```python
from build123d import *

# Parameters (mm, degrees)
F0_R     = 40.1
F1_DEPTH = 10
F2_R     = 38.1
F3_DEPTH = 8
F4_R     = 0.99999


# Not quite as in the source:
# - a fillet or chamfer is up to 0.001 mm smaller than in the source, because OpenCascade refuses the exact size


with BuildPart() as f1:
    # F0 (on Top) → F1 (new body)
    with BuildSketch(Plane.XY):
        Circle(F0_R)
    extrude(amount=F1_DEPTH)

    # F2 (on face) → F3 (cut)
    with BuildSketch(Plane.XY.offset(10)):
        Circle(F2_R)
    extrude(amount=-F3_DEPTH, mode=Mode.SUBTRACT)

    # F4 (radius 1 in the source; OpenCascade refuses exactly that, so slightly less here)
    f4_edges = [f1.edges().sort_by_distance(p)[0] for p in [
        (-38.1, 0, 10),
        (-40.1, 0, 10),
    ]]
    fillet(f4_edges, radius=F4_R)


solid = f1.part
```
The listing builds one solid part. Answer for the finished solid, in the listing's coordinates (mm). Give positions to 0.01 mm unless a question says otherwise; leave off trailing zeros. Order: outer loops, then holes, each group sorted by start corner. A loop starts at its lowest first (then second) coordinate and runs counter-clockwise, first axis right, second up.
1) Find section C-C on z = 6. Write down the section's boundary in (x, y).
Reported:
outline: circle Ø80.2 at (0, 0); hole circle Ø76.2 at (0, 0)
2) Consider line 1 along Y through (x, z) = (0, 4.25); line 2 along Z through (x, y) = (1.5, -9.5); line 3 along X through (y, z) = (-22.5, 4). Determine where each line is inside the solid, lowest interval first.
Reported:
line 1: y = -40.1 to -38.1, 38.1 to 40.1
line 2: z = 0 to 2
line 3: x = -33.19 to -30.75, 30.75 to 33.19
3) Given P1, Ø2, axis at x = 8.5, y = 16.5, coming from the +Z side; P2, Ø3, axis at y = -8.5, z = 2, coming from the +X side; P3, Ø6, axis at y = -9, z = 3, coming from the +X side, each flat-ended and moving along its own axis, determine where each tip first touches the part or whether it passes through.
Reported:
P1: stops at z = 2
P2: stops at x = 39.48
P3: stops at x = 39.65
4) Determine the mould class of faces 1 (the face through (-30.235, -23.183, 5.549)), 2 (the face through (-1, 1, 0)), 3 (the face through (-31.82, -24.4, 4.44)), 4 (the face through (-1, 1, 2)) for opening direction Y: pulls with the +Y half, pulls with the -Y half, needs draft (parallel to the pull), parting line crosses it, or undercut.
Reported:
face 1: undercut
face 2: needs draft
face 3: parting line crosses it
face 4: undercut
